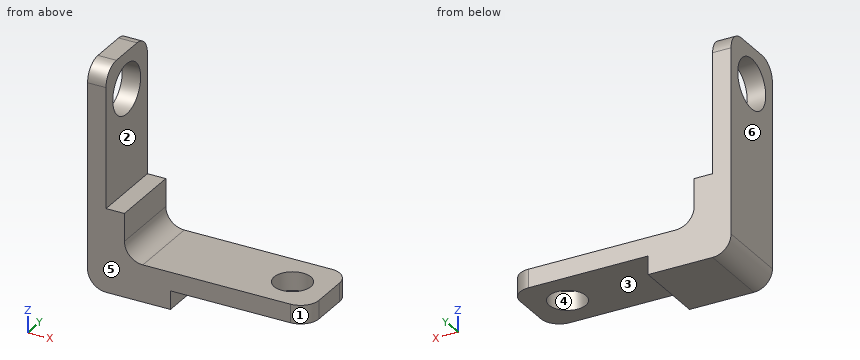
from build123d import *

# Parameters (mm, degrees)
SKETCH2_W           = 120
SKETCH2_H           = 40
BOSS_EXTRUDE1_DEPTH = 20
SKETCH3_W           = 20
SKETCH3_H           = 40
BOSS_EXTRUDE2_DEPTH = 100
SKETCH4_W           = 75
SKETCH4_H           = 40
CUT_EXTRUDE1_DEPTH  = 10
SKETCH5_W           = 75
SKETCH5_H           = 40
CUT_EXTRUDE2_DEPTH  = 10
CUT_EXTRUDE3_REACH  = 12
SKETCH6_R           = 13.5
FILLET2_R           = 10
SKETCH7_R           = 10
CUT_EXTRUDE4_DEPTH  = 10
FILLET3_R           = 10


with BuildPart() as part:
    # Sketch2 → Boss-Extrude1 (new body)
    with BuildSketch(Plane.XY):
        Rectangle(SKETCH2_W, SKETCH2_H)
    extrude(amount=BOSS_EXTRUDE1_DEPTH)

    # Sketch3 → Boss-Extrude2 (add)
    with BuildSketch(Plane.XY.offset(20)):
        with Locations((-50, 0)):
            Rectangle(SKETCH3_W, SKETCH3_H)
    extrude(amount=BOSS_EXTRUDE2_DEPTH)

    # Sketch4 → Cut-Extrude1 (cut)
    with BuildSketch(Plane(origin=(0, 0, 0), x_dir=(-1, 0, 0), z_dir=(0, 0, -1))):
        with Locations((-22.5, 0)):
            Rectangle(SKETCH4_W, SKETCH4_H)
    extrude(amount=-CUT_EXTRUDE1_DEPTH, mode=Mode.SUBTRACT)

    # Sketch5 → Cut-Extrude2 (cut)
    with BuildSketch(Plane(origin=(-40, 0, 0), x_dir=(0, 0, -1), z_dir=(1, 0, 0))):
        with Locations((-82.5, 0)):
            Rectangle(SKETCH5_W, SKETCH5_H)
    extrude(amount=-CUT_EXTRUDE2_DEPTH, mode=Mode.SUBTRACT)

    # Sketch6 → Cut-Extrude3 (cut, up to next)
    with BuildSketch(Plane(origin=(-50, 0, 0), x_dir=(0, 0, -1), z_dir=(1, 0, 0)), mode=Mode.PRIVATE) as cut_extrude3_sk1:
        with Locations((-100, 0)):
            Circle(SKETCH6_R)
    cut_extrude3_tool1 = extrude(cut_extrude3_sk1.sketch, amount=-CUT_EXTRUDE3_REACH, mode=Mode.PRIVATE) & part.part
    add(cut_extrude3_tool1.solids().sort_by_distance((-50, 0, 100))[0], mode=Mode.SUBTRACT)

    # Fillet2
    fillet2_edges = [part.edges().sort_by_distance(p)[0] for p in [
        (60, 20, 15),
        (60, -20, 15),
        (-55, -20, 120),
        (-55, 20, 120),
        (-60, 0, 0),
    ]]
    fillet(fillet2_edges, radius=FILLET2_R)

    # Sketch7 → Cut-Extrude4 (cut)
    with BuildSketch(Plane.XY.offset(20)):
        with Locations((40, 0)):
            Circle(SKETCH7_R)
    extrude(amount=-CUT_EXTRUDE4_DEPTH, mode=Mode.SUBTRACT)

    # Fillet3
    fillet3_edges = [part.edges().sort_by_distance(p)[0] for p in [
        (-40, 0, 20),
    ]]
    fillet(fillet3_edges, radius=FILLET3_R)


solid = part.part
CAD build for the part. Positions are in the model's coordinates, mm. Face numbers are marked on the shaded views. A direction names the side the tool comes from. Coordinates: 2 decimals unless noted, no trailing zeros. Write each loop counter-clockwise with the first axis right and the second up, starting at its lowest first coordinate (ties: lowest second). Pieces come first, ordered by that corner, then holes. Notation, with made-up numbers: (85.25, 86.25) - (112.25, 86.25) arc R27 cw to (112.25, 113.25) - close; hole circle Ø10 at (56.25, 84.25). An arc over 180 degrees is marked (long way). Use a Markdown table: item, result. Add a question column.
Item 1: Band-saw the part on D-D, the plane y = 0. Give the cut face in (x, z).
Item 2: Mould opens along X. For the marked faces 4, 5 and 6 say: pulls with the +X half, pulls with the -X half, needs draft (parallel to the pull), parting line crosses it, or undercut.
Item 3: 3-axis set-ups, long thin cutter, end or side, ignore diameter. For the marked faces 1, 2 and 3: which of +Z, -Z, +X, -X, +Y, -Y reach the whole face in a straight line?
Item 4: Band-saw the part on C-C, the plane x = 40. Give the cut face in (y, z), and give its area (3 significant figures).
Item 5: Flat gauge pins, fed straight in: pin 1 (1.5 mm diameter, centred on y = 0, z = 28, fed in from +X); pin 2 (20 mm diameter, centred on y = 7, z = 93, fed in from +X); pin 3 (20 mm diameter, centred on x = 12, y = 3.5, fed in from -Z). Where does each tip first touch, or does it go through?
Item 6: Band-saw the part on A-A, the plane z = 100. Give the cut face in (x, y), and give its area (3 significant figures).
Item 7: Drill centre lines: L1, parallel to Y at x = -53, z = 100; L2, parallel to Y at x = 40, z = 17; L3, parallel to Z at x = 35.5, y = -15.5. Where is each one in solid material? Low to high. Write a range as from..to.
Item 8: Band-saw the part on B-B, the plane z = 17.5. Give the cut face in (x, y), and give its area (3 significant figures).
Numbers:
| question | item | result |
|---|---|---|
| 1 | outline | (-60, 10) arc R10 ccw to (-50, 0) - (-15, 0) - (-15, 10) - (30, 10) - (30, 20) - (-30, 20) arc R10 cw to (-40, 30) - (-40, 45) - (-50, 45) - (-50, 86.5) - (-60, 86.5) - close; (-60, 113.5) - (-50, 113.5) - (-50, 120) - (-60, 120) - close; (50, 10) - (60, 10) - (60, 20) - (50, 20) - close |
| 2 | face 4 | undercut |
| 2 | face 5 | needs draft |
| 2 | face 6 | pulls with the -X half |
| 3 | face 1 | +Z, -Z, +X, -Y |
| 3 | face 2 | +Z, +X, +Y, -Y |
| 3 | face 3 | -Z, +X, +Y, -Y |
| 4 | outline | (-20, 10) - (-10, 10) - (-10, 20) - (-20, 20) - close; (10, 10) - (20, 10) - (20, 20) - (10, 20) - close |
| 4 | area | 200 mm2 |
| 5 | pin 1 | x = -39.61 |
| 5 | pin 2 | x = -50 |
| 5 | pin 3 | z = 10 |
| 6 | outline | (-60, -20) - (-50, -20) - (-50, -13.5) - (-60, -13.5) - close; (-60, 13.5) - (-50, 13.5) - (-50, 20) - (-60, 20) - close |
| 6 | area | 130 mm2 |
| 7 | L1 | -20..-13.5, 13.5..20 |
| 7 | L2 | -20..-10, 10..20 |
| 7 | L3 | 10..20 |
| 8 | outline | (-60, -20) - (50, -20) arc R10 ccw to (60, -10) - (60, 10) arc R10 ccw to (50, 20) - (-60, 20) - close; hole circle Ø20 at (40, 0) |
| 8 | area | 4,440 mm2 |
